Autodesk Inventor part; units mm, degrees
ref_plane "Work Plane9" through (67.562, 43.9221, 32.5482) normal (0, -1, 0) x (1, 0, 0)
ref_plane "Work Plane10" through (13.3602, 50.0901, 21.2671) normal (-0.003, 1, 0) x (0, 0, 1)
ref_plane "YZ Plane" through (0, 0, 0) normal (1, 0, 0) x (0, 1, 0)
ref_plane "Work Plane5" through (13.4046, 50.1721, 72.2727) normal (0, 1, 0) x (1, 0, 0)
sketch "Sketch7" plane through (13.4046, 50.1721, 72.2727) normal (0, 1, 0) x (1, 0, 0)
  circle A0 centre (6.5, 6.5) radius 2.5 construction
  circle A1 centre (48.5, 6.5) radius 2.5 construction
  line L0 (55, 2) -> (55, 11) construction
  line L1 (55, 35) -> (55, 44) construction
  circle A2 centre (48.5, 39.5) radius 2.5 construction
  circle A3 centre (6.5, 39.5) radius 2.5 construction
  line L2 (0, 35) -> (0, 44) construction
  line L3 (16.5, 85.8) -> (16.5, 84) construction
  line L4 (38.5, 85.8) -> (38.5, 84) construction
  line L5 (38.5, 84) -> (16.5, 84) construction
  line L6 (2, 0) -> (53, 0) construction
  line L7 (0, 38.8) -> (55, 38.8)
  line L8 (55, 38.8) -> (55, 85.8)
  line L9 (55, 85.8) -> (0, 85.8)
  line L10 (0, 85.8) -> (0, 38.8)
  line L11 (0, 85.8) -> (55, 85.8)
  line L12 (55, 85.8) -> (55, 89.8)
  line L13 (55, 89.8) -> (0, 89.8)
  line L14 (0, 89.8) -> (0, 85.8)
  point P0 (-13.4046, 72.2727)
  dimension "d112" = 47
  dimension "d115" = 4
extrude "Extrusion7" add sketch "Sketch7" along normal blind 16
sketch "Sketch8" plane through (13.4046, 50.1721, -13.5273) normal (-1, 0, 0) x (0, 0, 1)
  circle A0 centre (50.2042, 7.5) radius 2.3
  circle A1 centre (30.4132, 7.5) radius 6
  point P0 (13.5273, -50.1721)
  dimension "d77" = 12
extrude "Extrusion8" cut sketch "Sketch8" against normal through all contours A1
sketch "Sketch9" plane through (13.4046, 50.1721, 72.2727) normal (0, -1, 0) x (1, 0, 0)
  circle A0 centre (48.5, -44.5) radius 2.5
  circle A1 centre (6.5, -44.5) radius 2.5
  ellipse E0 centre (6.4724, -21.5) end of major axis (6.4724, -19) minor radius 2.5
  ellipse E1 centre (48.4722, -21.5) end of major axis (48.4722, -19) minor radius 2.5
  point P0 (-13.4046, -72.2727)
  point P1 (6.5, -6.5)
  point P2 (48.5, -6.5)
hole "Hole1" at (19.9046, 50.1721, 65.7727) at (61.9046, 50.1721, 65.7727) at (61.9046, 50.1721, 27.7727) at (19.9046, 50.1721, 27.7727) at (61.8768, 50.1721, 50.7727) at (19.877, 50.1721, 50.7727) direction (0, 1, 0) diameter 2.9 end through all
sketch "Sketch10" plane through (68.4046, 50.1721, -17.5273) normal (0, 0, -1) x (-1, 0, 0)
  circle A0 centre (39, -26) radius 1
  circle A1 centre (16, -26) radius 1
  circle A2 centre (16, -3) radius 1
  circle A3 centre (39, -3) radius 1.1
  circle A4 centre (27.5, -14.5) radius 12
  circle A5 centre (27.5, -14.5) radius 10.8
  line L0 (55, 0) -> (0, 0)
  line L1 (11.5, -29) -> (43.5, -29)
  line L2 (43.5, -29) -> (43.5, 0)
  line L3 (43.5, 0) -> (11.5, 0)
  line L4 (11.5, 0) -> (11.5, -29)
  line L5 (11.5, -29) -> (43.5, 0) construction
  line L6 (43.5, -29) -> (11.5, 0) construction
  line L7 (0, 0) -> (11.5, 0)
  line L8 (43.5, 0) -> (55, 0)
  line L9 (55, 0) -> (43.5, 0)
  line L10 (43.5, 0) -> (43.5, -29)
  line L11 (43.5, -29) -> (55, -29)
  line L12 (55, -29) -> (55, 0)
  line L13 (11.5, -29) -> (0, -29)
  line L14 (0, -29) -> (0, 0)
  line L15 (0, 0) -> (11.5, 0)
  line L16 (11.5, 0) -> (11.5, -29)
  circle A6 centre (47.5, -14.5) radius 3 construction
  circle A7 centre (7.5, -14.5) radius 3 construction
  circle A8 centre (47.5, -14.5) radius 3.1
  circle A9 centre (7.5, -14.5) radius 3.1
  line L17 (21.9985, -30) -> (32.9661, -30)
  line L18 (55, -29) -> (0, -29)
  line L19 (0, -29) -> (0, -30)
  line L20 (0, -30) -> (55, -30)
  line L21 (55, -30) -> (55, -29)
  point P0 (68.4046, -50.1721)
  dimension "d50" = 24
  dimension "d51" = 32
  dimension "d67" = 6.2
  dimension "d68" = 6.2
extrude "Extrusion9" add sketch "Sketch10" against normal blind 10 contours L12 L11 L2 L0 | L2 L1 L4 L0 | L21 L20 L17 L19 L13 L1 L11 | L4 L13 L14 L0 | A8 | A9
sketch "Sketch15" plane through (68.4046, 50.1721, 33.4727) normal (1, 0, 0) x (0, 0, -1)
  line L0 (41, 0) -> (0, 0)
  line L1 (0, 16) -> (51, 16)
  line L2 (0, 0) -> (0, 16)
  line L3 (51, 16) -> (0, 16)
  line L4 (28, 16) -> (0, 16)
  line L5 (0, 16) -> (0, 7)
  line L6 (0, 7) -> (28, 7)
  line L7 (51, 9) -> (44.5, 9) construction
  line L8 (24.9, 18.4) -> (24.9, 10.6) construction
  line L9 (55.3238, 21.5045) -> (24.6, 21.5045)
  line L10 (24.6, 21.5045) -> (24.6, 8.9)
  line L11 (24.6, 8.9) -> (55.3238, 8.9)
  line L12 (55.3238, 8.9) -> (55.3238, 21.5045)
  line L13 (51, -30) -> (51, 16)
  line L14 (41, -30) -> (41, 0)
  line L15 (51, -30) -> (41, -30)
  point P0 (33.4727, -50.1721)
  point P1 (47, 16)
  dimension "d73" = 7
  dimension "d113" = 0.1
  dimension "d114" = 0.3
extrude "Extrusion12" cut sketch "Sketch15" against normal through all contours L13 L1 L10 L9 L12 L11 | L11 L10 L1 L13
sketch "Sketch17" plane through (13.4046, 50.1721, 72.2727) normal (0, -1, 0) x (1, 0, 0)
  circle A0 centre (37.5, -66.9) radius 1.5
  circle A1 centre (17.5, -66.9) radius 1.25
  circle A2 centre (17.5, -86.9) radius 1.25
  circle A3 centre (37.5, -86.9) radius 1.25
  point P0 (-13.4046, -72.2727)
hole "Hole4" at (50.9046, 50.1721, 5.3727) at (30.9046, 50.1721, 5.3727) direction (0, 1, 0) diameter 3.5 end through all counterbore diameter 7 counterbore depth 4
ref_plane "Work Plane8" through (68.4046, 50.1721, 12.4727) normal (0, 0, 1) x (1, 0, 0)
sketch "Sketch18" plane through (68.4046, 50.1721, 12.4727) normal (0, 0, 1) x (1, 0, 0)
  circle A0 centre (-27.5, -14.5) radius 12
  circle A1 centre (-39, -3) radius 1.1
  circle A2 centre (-16, -3) radius 1
  circle A3 centre (-16, -26) radius 1
  circle A4 centre (-39, -26) radius 1
  line L0 (0, -30) -> (0, 0)
  line L1 (-55, 0) -> (0, 0)
  line L2 (-55, 0) -> (-55, -30)
  line L3 (-55, -30) -> (0, -30)
  point P0 (-68.4046, -50.1721)
extrude "Extrusion13" add sketch "Sketch18" along normal blind 6 and the other way blind 3
sketch "Sketch23" plane through (13.4046, 50.1721, 33.4727) normal (-1, 0, 0) x (0, 0, 1)
  line L0 (-24.6, 8.9) -> (-51, 8.9)
  line L1 (-51, 8.9) -> (-51, -30)
  line L2 (-41, 0) -> (-41, -30)
  line L3 (-24, 0) -> (-41, 0)
  line L4 (0, 0) -> (0, 16)
  line L5 (-24.6, 16) -> (0, 16)
  line L6 (-24.6, 16) -> (-24.6, 8.9)
  circle A0 centre (-16.5868, 7.5) radius 6
  line L7 (-24.6, 16) -> (-51, 16)
  line L8 (-51, 16) -> (-51, 8.9)
  line L9 (-51, 8.9) -> (-24.6, 8.9)
  line L10 (-24.6, 8.9) -> (-24.6, 16)
  line L11 (-31.1222, 16) -> (-45.0868, 16)
  line L12 (-45.0868, 16) -> (-45.0868, 13)
  line L13 (-45.0868, 13) -> (-31.1222, 13)
  line L14 (-31.1222, 13) -> (-31.1222, 16)
  line L15 (-32.6207, 14) -> (-43.5883, 14)
  line L16 (-32.1222, 15.1785) -> (-32.1221, 14.4985)
  line L17 (-43.5883, 14) -> (-44.0868, 14.4985)
  circle A1 centre (-31.2, 11.995) radius 2.1 construction
  circle A2 centre (-45, 11.995) radius 2.1 construction
  line L18 (-24, -30) -> (-24, 0)
  line L19 (-15, 0) -> (-15, -30)
  line L20 (0, 0) -> (-15, 0)
  line L21 (-51, -30) -> (-41, -30)
  line L22 (-15, -30) -> (-24, -30)
  point P0 (-33.4727, -50.1721)
  dimension "d116" = 1
  dimension "d117" = 1
  dimension "d118" = 1
extrude "Extrusion18" add sketch "Sketch23" against normal blind 3 contours L0 L8 L7 L12 L13 L14 L6
sketch "Sketch24" plane through (13.4046, 50.1721, 33.4727) normal (-1, 0, 0) x (0, 0, 1)
  circle A0 centre (-45, 11.995) radius 2.1
  circle A1 centre (-31.2, 11.995) radius 2.1
  circle A2 centre (-38.1, 11.995) radius 1.5
  point P0 (-33.4727, -50.1721)
  dimension "d121" = 3
  dimension "d122" = 6.9
extrude "Extrusion19" cut sketch "Sketch24" against normal through all contours A2
sketch "Sketch25" plane through (68.4046, 50.1721, 33.4727) normal (1, 0, 0) x (0, 0, -1)
  circle A0 centre (16.5868, 7.5) radius 6
  arc A1 (36.9865, 13) -> (39.2136, 13) centre (38.1, 11.995) ccw
  line L0 (39.2136, 13) -> (45.0868, 13)
  line L1 (45.0868, 13) -> (45.0868, 16)
  line L2 (45.0868, 16) -> (51, 16)
  line L3 (51, 16) -> (51, -30)
  line L4 (41, 0) -> (41, -30)
  line L5 (24, 0) -> (41, 0)
  line L6 (0, 0) -> (0, 16)
  line L7 (31.1222, 16) -> (0, 16)
  line L8 (31.1222, 16) -> (31.1222, 13)
  line L9 (31.1222, 13) -> (36.9865, 13)
  line L10 (51, 8.9) -> (47.0344, 8.9)
  line L11 (51, 8.9) -> (24.5983, 8.9)
  line L12 (24.5983, 8.9) -> (24.5983, 16)
  line L13 (24, -30) -> (24, 0)
  line L14 (15, 0) -> (15, -30)
  line L15 (0, 0) -> (15, 0)
  line L16 (51, -30) -> (41, -30)
  line L17 (15, -30) -> (24, -30)
  point P0 (33.4727, -50.1721)
extrude "Extrusion20" add sketch "Sketch25" against normal blind 3 contours A1 L0 L1 L2 L3 L10 L11 L12 L7 L8 L9
sketch "Sketch26" plane through (68.4046, 50.1721, 33.4727) normal (1, 0, 0) x (0, 0, -1)
  circle A0 centre (24.5868, 7.5) radius 1.625
  circle A1 centre (8.5868, 7.5) radius 1.625
  point P0 (33.4727, -50.1721)
hole "Hole5" at (68.4046, 57.6721, 8.8859) at (68.4046, 57.6721, 24.8859) direction (-1, 0, 0) diameter 2.8 end through all
sketch "Sketch28" plane through (68.4046, 50.1721, 18.4727) normal (0, 0, 1) x (1, 0, 0)
  circle A0 centre (-27.5, -14.5) radius 12
  circle A1 centre (-39, -3) radius 1.1
  circle A2 centre (-39, -26) radius 1
  circle A3 centre (-16, -26) radius 1
  circle A4 centre (-16, -3) radius 1
  line L0 (0, -30) -> (0, 0)
  line L1 (-55, 0) -> (0, 0)
  line L2 (-55, 0) -> (-55, -30)
  line L3 (-55, -30) -> (0, -30)
  point P0 (-68.4046, -50.1721)
hole "Hole7" at (52.4046, 24.1721, 18.4727) at (29.4046, 24.1721, 18.4727) at (29.4046, 47.1721, 18.4727) at (52.4046, 47.1721, 18.4727) direction (0, 0, -1) diameter 4 depth 8 tip angle 118
sketch "Sketch29" plane through (13.4046, 20.1721, -17.5273) normal (0, -1, 0) x (1, 0, 0)
  line L0 (0, 0) -> (55, 0)
  line L1 (55, 0) -> (55, 10)
  line L2 (0, 10) -> (55, 10)
  line L3 (0, 0) -> (0, 10)
  line L4 (55, 36) -> (55, 27)
  line L5 (0, 36) -> (55, 36)
  line L6 (0, 36) -> (0, 27)
  line L7 (55, 27) -> (0, 27)
  arc A0 (29.113, 42.4017) -> (29.113, 40.9628) centre (27.5177, 41.6823) ccw
  circle A1 centre (27.5177, 31.5) radius 1.4
  circle A2 centre (27.5177, 6.5) radius 1.4
  line L8 (50.0177, 6.5) -> (5.0177, 6.5)
  line L9 (5.0177, 6.5) -> (5.0177, 31.5)
  line L10 (5.0177, 31.5) -> (50.0177, 31.5)
  line L11 (50.0177, 31.5) -> (50.0177, 6.5)
  line L12 (50.0177, 6.5) -> (5.0177, 31.5) construction
  line L13 (5.0177, 6.5) -> (50.0177, 31.5) construction
  point P0 (-13.4046, 17.5273)
  point P1 (27.5177, 19)
  dimension "d150" = 2.8
  dimension "d151" = 2.8
  dimension "d152" = 45
  dimension "d153" = 25
hole "Hole8" at (18.4223, 20.1721, 13.9727) at (40.9223, 20.1721, 13.9727) at (63.4223, 20.1721, 13.9727) at (63.4223, 20.1721, -11.0273) at (40.9223, 20.1721, -11.0273) at (18.4223, 20.1721, -11.0273) direction (0, 1, 0) diameter 2.8 depth 8 tip angle 118
sketch "Sketch30" plane through (13.4046, 50.1721, 72.2727) normal (0, -1, 0) x (1, 0, 0)
  circle A0 centre (6.5, -44.5) radius 1.45
  circle A1 centre (48.5, -44.5) radius 1.45
  line L0 (0, -53.8) -> (55, -53.8)
  line L1 (55, -53.8) -> (55, -38.8)
  line L2 (0, -38.8) -> (55, -38.8)
  line L3 (0, -38.8) -> (0, -53.8)
  line L4 (55, -53.8) -> (55, -38.8)
  line L5 (55, -42.175) -> (60, -42.175)
  line L6 (60, -42.175) -> (60, -40.175)
  line L7 (60, -40.175) -> (55, -40.175)
  line L8 (55, -40.175) -> (55, -42.175)
  point P0 (-13.4046, -72.2727)
  dimension "d161" = 5
  dimension "d162" = 2
ref_plane "Work Plane9" through (67.562, 43.9221, 32.5482) normal (0, -1, 0) x (1, 0, 0)
extrude "Extrusion21" add sketch "Sketch30" against normal up to surface (22.25 mm away) from surface at 6.25 contours L1 L7 L6 L5
sketch "Sketch31" plane through (13.4046, 66.1721, 72.2727) normal (0, 1, 0) x (1, 0, 0)
  circle A0 centre (48.5, 44.5) radius 1.45
  circle A1 centre (6.5, 44.5) radius 1.45
  line L0 (55, 38.8) -> (55, 40.175)
  line L1 (60, 40.175) -> (55, 40.175)
  line L2 (60, 42.175) -> (60, 40.175)
  line L3 (55, 42.175) -> (60, 42.175)
  line L4 (55, 42.175) -> (55, 69.9222)
  line L5 (55, 69.9222) -> (52, 69.9222) construction
  line L6 (52, 63.4) -> (52, 69.9222) construction
  line L7 (52, 63.4) -> (3, 63.4)
  line L8 (3, 69.9222) -> (3, 63.4)
  line L9 (3, 69.9222) -> (0, 69.9222)
  line L10 (0, 69.9222) -> (0, 38.8)
  line L11 (0, 38.8) -> (55, 38.8)
  line L12 (60, 40.175) -> (55, 40.175)
  line L13 (0, 38.8) -> (55, 38.8)
  line L14 (60, 40.175) -> (55, 38.8)
  line L15 (55, 38.8) -> (55, 44.5)
  line L16 (55, 42.175) -> (60, 42.175)
  line L17 (60, 42.175) -> (55, 44.2246)
  point P0 (-13.4046, 72.2727)
ref_plane "Work Plane10" through (13.3602, 50.0901, 21.2671) normal (-0.003, 1, 0) x (0, 0, 1)
extrude "Extrusion22" add sketch "Sketch31" against normal up to surface contours L0 L1 L14 | L15 L3 L2 L1 | L4 L17 L3 surface through (13.3602, 50.0901, 21.2671) normal (-0.003, 1, 0)
sketch "Sketch32" plane through (68.4046, 20.1721, -17.5273) normal (0, 0, -1) x (-1, 0, 0)
  line L0 (52, 38.9) -> (3, 38.9)
  line L1 (3, 46) -> (3, 38.9)
  line L2 (0, 46) -> (3, 46)
  line L3 (0, 0) -> (0, 46)
  line L4 (55, 0) -> (0, 0)
  line L5 (55, 46) -> (55, 0)
  line L6 (55, 46) -> (52, 46)
  line L7 (52, 38.9) -> (52, 46)
  circle A0 centre (39, 4) radius 1
  circle A1 centre (16, 4) radius 1
  circle A2 centre (16, 27) radius 1
  circle A3 centre (39, 27) radius 1.1
  circle A4 centre (27.5, 15.5) radius 12
  point P0 (68.4046, -20.1721)
hole "Hole9" at (29.4046, 47.1721, -17.5273) at (29.4046, 24.1721, -17.5273) at (52.4046, 24.1721, -17.5273) at (52.4046, 47.1721, -17.5273) direction (0, 0, 1) diameter 2.5 end through all
properties part number "01_Slide_camera_x_v0"
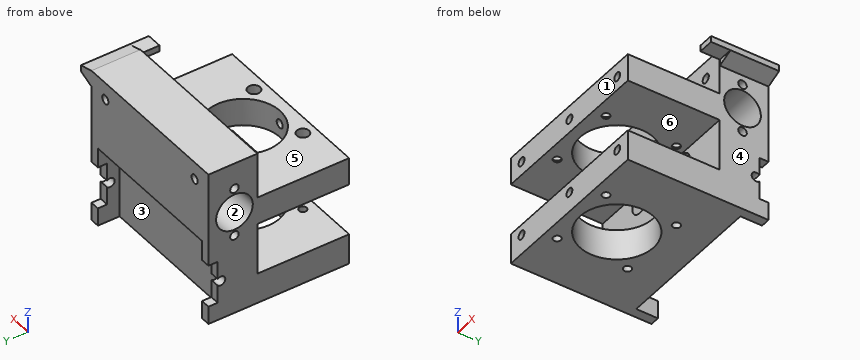
Could you check a few things on this model? Use its own coordinates, in mm. Face numbers are marked on the shaded views. A direction names the side the tool comes from. Coordinates: 2 decimals unless noted, no trailing zeros. Order: outer loops, then holes, each group sorted by start corner. A loop starts at its lowest first (then second) coordinate and runs counter-clockwise, first axis right, second up. Notation, with made-up numbers: M 4,-6 L 31,-6 A20 ccw 31,24 Z; hole C 49,-0.5 d10. An arc over 180 degrees is marked long. Use a Markdown table: item, result. Add a question column.
Q1. I want a section at B-B on x = 44. List the corners of the cut face in (y, z) for me.
Q2. I want a section at D-D on y = 30.5. List the corners of the cut face in (x, z) for me.
Q3. Which directions (+Z, -Z, +X, -X, +Y, -Y) give clear straight access to the entire face, cutting with the end or side of a thin tool? Please do the marked faces 4, 5 and 6.
Q4. I want a section at C-C on z = 16.5. List the corners of the cut face in (x, y) for me.
Q5. We'd pull the mould along Y, two halves only. Please class the marked faces 1, 2 and 3: pulls with the +Y half, pulls with the -Y half, needs draft (parallel to the pull), parting line crosses it, or undercut.
Q6. I want a section at A-A on y = 61.5. List the corners of the cut face in (x, z) for me, then the cut area to 3 significant figures.
Q7. I'm going to push flat-ended pins straight in: pin 1 (3 mm diameter, centred on x = 58.5, z = -2, fed in from +Y); pin 2 (3 mm diameter, centred on x = 52.4, y = 47.17, fed in from +Z); pin 3 (2 mm diameter, centred on y = 49.5, z = 26, fed in from +X). Where does each tip first touch, or does it pass through?
Q8. If I drill on L1, parallel to Z at x = 29, y = 40.5; L2, parallel to X at y = 54, z = 7.5; L3, parallel to Y at x = 30.5, z = 17.5, over which ranges is the centre line in solid material (lowest first)?
Checked values:
| question | item | result |
|---|---|---|
| 1 | outline | M 20.17,-17.53 L 24.08,-17.53 L 24.08,-7.53 L 20.17,-7.53 Z; M 20.17,9.47 L 24.08,9.47 L 24.08,18.47 L 20.17,18.47 Z; M 47.27,-17.53 L 59.07,-17.53 L 59.07,8.87 L 66.17,8.87 L 66.17,33.47 L 50.17,33.47 L 50.17,18.47 L 47.27,18.47 L 47.27,9.47 L 50.17,9.47 L 50.17,-7.53 L 47.27,-7.53 Z; hole C 57.67,16.89 d12; hole C 57.67,8.89 d2.8; hole C 57.67,24.89 d2.8 |
| 2 | outline | M 13.4,-17.53 L 30.08,-17.53 L 30.08,-7.53 L 13.4,-7.53 Z; M 13.4,9.47 L 30.08,9.47 L 30.08,18.47 L 13.4,18.47 Z; M 51.73,-17.53 L 68.4,-17.53 L 68.4,-7.53 L 51.73,-7.53 Z; M 51.73,9.47 L 68.4,9.47 L 68.4,18.47 L 51.73,18.47 Z |
| 3 | face 4 | -Z, +X, +Y, -Y |
| 3 | face 5 | +Z, +X, -X, -Y |
| 3 | face 6 | +X, -X, -Y |
| 4 | outline | M 13.4,20.17 L 68.4,20.17 L 68.4,51.68 L 13.4,51.68 Z; M 13.4,63.66 L 68.4,63.66 L 68.4,66.17 L 13.4,66.17 Z; hole C 29.4,24.17 d4; hole C 29.4,47.17 d4; hole C 40.9,35.67 d24; hole C 52.4,24.17 d4; hole C 52.4,47.17 d4 |
| 5 | face 1 | pulls with the -Y half |
| 5 | face 2 | undercut |
| 5 | face 3 | pulls with the +Y half |
| 6 | outline | M 13.4,-17.53 L 16.4,-17.53 L 16.4,-5.97 L 13.4,-5.97 Z; M 13.4,-3.28 L 16.4,-3.28 L 16.4,8.87 L 65.4,8.87 L 65.4,-3.28 L 68.4,-3.28 L 68.4,12.27 L 13.4,12.27 Z; M 13.4,21.51 L 68.4,21.51 L 68.4,28.05 L 73.4,30.1 L 73.4,32.1 L 68.4,33.47 L 13.4,33.47 Z; M 65.4,-17.53 L 68.4,-17.53 L 68.4,-5.97 L 65.4,-5.97 Z; hole C 19.9,27.77 d2.9; hole C 61.9,27.77 d2.9 |
| 6 | area | 992 mm² |
| 7 | pin 1 | y = 59.07 |
| 7 | pin 2 | z = 10.18 |
| 7 | pin 3 | x = 68.4 |
| 8 | L1 | -17.53 to -7.53, 9.47 to 18.47 |
| 8 | L2 | 13.4 to 28.13, 33.68 to 48.13, 53.68 to 68.4 |
| 8 | L3 | 20.17 to 22.5, 25.85 to 29.69, 41.65 to 45.5, 48.85 to 51.7, 63.64 to 66.17 |
